Could you check a few things on this model? Use its own coordinates, in mm. Give positions to 0.01 mm unless a question says otherwise; leave off trailing zeros. Loops run counter-clockwise (first coordinate to the right, second up) from the corner with the lowest first, then second, coordinate; pieces in that order, holes last. Notation, with made-up numbers: M 53,79 L 73,79 A23 cw 73,112 Z; hole C 72.25,-37.75 d10. An arc over 180 degrees is marked long. Answer in a Markdown table with one row per item. Add a question column.
1. If we section it at D-D on x = -15.5: List the corners of the cut face in (y, z) for me.
2. Thinking about a two-plate mould opening in X: for faces 1 (the cylindrical face through (-2.539, 19.334, 1.479)), 2 (the flat face through (0, 5, 3)), 3 (the cylindrical face through (13.9, -1.2, 1.5)), which applies, released by +X, released by -X, zero draft, split by the parting line, or undercut?
3. If we section it at C-C on z = 0.5: List the corners of the cut face in (x, y) for me, then the cut area to 3 significant figures.
4. I need wall thicknesses on line 1 along Y through (x, z) = (0, 1.55); line 2 along X through (y, z) = (-1, 2.35); line 3 along X through (y, z) = (-0.5, 2.7). Which ranges of each line are inside material? Lowest first, please. Write a range as from..to.
5. I'm going to push flat-ended pins straight in: pin 1 Ø1 at (x, z) = (11, 1) entering from +Y; pin 2 Ø7 at (x, y) = (0, 0) entering from +Z; pin 3 Ø1 at (x, z) = (-2.5, 1.5) entering from -Y. Where does each tip first touch, or does it pass through?
6. If we section it at A-A on x = 0: List the corners of the cut face in (y, z) for me.
```python
from build123d import *

# Parameters (mm, degrees)
CROQUIS1_R              = 19.5
CROQUIS1_R_2            = 2
SALIENTE_EXTRUIR1_DEPTH = 3
CROQUIS4_R              = 4.5
CORTAR_EXTRUIR1_DEPTH   = 1
CROQUIS4_2_R            = 4.5
CORTAR_EXTRUIR2_DEPTH   = 3


with BuildPart() as part:
    # Croquis1 → Saliente-Extruir1 (new body)
    with BuildSketch(Plane.XY):
        Circle(CROQUIS1_R)
        with Locations((0, -15.5)):
            Circle(CROQUIS1_R_2, mode=Mode.SUBTRACT)
        with Locations((15.5, 0)):
            Circle(CROQUIS1_R_2, mode=Mode.SUBTRACT)
        with Locations((0, 15.5)):
            Circle(CROQUIS1_R_2, mode=Mode.SUBTRACT)
        with Locations((-15.5, 0)):
            Circle(CROQUIS1_R_2, mode=Mode.SUBTRACT)
    extrude(amount=SALIENTE_EXTRUIR1_DEPTH)

    # Croquis4 → Cortar-Extruir1 (cut)
    with BuildSketch(Plane(origin=(0, 0, 0), x_dir=(-1, 0, 0), z_dir=(0, 0, -1))):
        Circle(CROQUIS4_R)
    extrude(amount=-CORTAR_EXTRUIR1_DEPTH, mode=Mode.SUBTRACT)

    # Croquis4<2> → Cortar-Extruir2 (cut)
    with BuildSketch(Plane(origin=(0, 0, 0), x_dir=(-1, 0, 0), z_dir=(0, 0, -1))):
        Circle(CROQUIS4_2_R)
    extrude(amount=-CORTAR_EXTRUIR2_DEPTH, mode=Mode.SUBTRACT)


solid = part.part
```
Results:
| question | item | result |
|---|---|---|
| 1 | outline | M -11.83,0 L -2,0 L -2,3 L -11.83,3 Z; M 2,0 L 11.83,0 L 11.83,3 L 2,3 Z |
| 2 | face 1 | split by the parting line |
| 2 | face 2 | zero draft |
| 2 | face 3 | undercut |
| 3 | outline | C 0,0 d39; hole C -15.5,0 d4; hole C 0,0 d9; hole C 0,-15.5 d4; hole C 0,15.5 d4; hole C 15.5,0 d4 |
| 3 | area | 1,080 mm2 |
| 4 | line 1 | -19.5..-17.5, -13.5..-4.5, 4.5..13.5, 17.5..19.5 |
| 4 | line 2 | -19.47..-17.23, -13.77..-4.39, 4.39..13.77, 17.23..19.47 |
| 4 | line 3 | -19.49..-17.44, -13.56..-4.47, 4.47..13.56, 17.44..19.49 |
| 5 | pin 1 | y = 16.43 |
| 5 | pin 2 | through |
| 5 | pin 3 | y = -19.4 |
| 6 | outline | M -19.5,0 L -17.5,0 L -17.5,3 L -19.5,3 Z; M -13.5,0 L -4.5,0 L -4.5,3 L -13.5,3 Z; M 4.5,0 L 13.5,0 L 13.5,3 L 4.5,3 Z; M 17.5,0 L 19.5,0 L 19.5,3 L 17.5,3 Z |
